```python
from build123d import *

# Parameters (mm, degrees)
ESBO_O1_W                = 23
ESBO_O1_H                = 38
ESBO_O1_W_2              = 15
ESBO_O1_H_2              = 30
RESSALTO_EXTRUS_O1_DEPTH = 3
CHANFRO1_SIZE            = 2
CHANFRO1_SIZE2           = 2.14473742
CHANFRO1_PART_2_SIZE     = 2
CHANFRO1_PART_2_SIZE2    = 2.14473742
CHANFRO1_PART_3_SIZE     = 2
CHANFRO1_PART_3_SIZE2    = 2.14473742
CHANFRO1_PART_4_SIZE     = 2
CHANFRO1_PART_4_SIZE2    = 2.14473742


with BuildPart() as part:
    # Esboço1 → Ressalto-extrusão1 (new body)
    with BuildSketch(Plane.XY):
        Rectangle(ESBO_O1_W, ESBO_O1_H)
        Rectangle(ESBO_O1_W_2, ESBO_O1_H_2, mode=Mode.SUBTRACT)
    extrude(amount=RESSALTO_EXTRUS_O1_DEPTH)

    # Chanfro1
    chanfro1_edges = [part.edges().sort_by_distance(p)[0] for p in [
        (11.5, 0, 3),
    ]]
    chanfro1_side = [part.faces().sort_by_distance(p)[0] for p in [
        (11.5, 0, 1.5),
    ]]
    chamfer(chanfro1_edges, length=CHANFRO1_SIZE, length2=CHANFRO1_SIZE2, reference=chanfro1_side[0])

    # Chanfro1 part 2
    chanfro1_part_2_edges = [part.edges().sort_by_distance(p)[0] for p in [
        (0, 19, 3),
    ]]
    chanfro1_part_2_side = [part.faces().sort_by_distance(p)[0] for p in [
        (0, 19, 1.5),
    ]]
    chamfer(chanfro1_part_2_edges, length=CHANFRO1_PART_2_SIZE, length2=CHANFRO1_PART_2_SIZE2, reference=chanfro1_part_2_side[0])

    # Chanfro1 part 3
    chanfro1_part_3_edges = [part.edges().sort_by_distance(p)[0] for p in [
        (-11.5, 0, 3),
    ]]
    chanfro1_part_3_side = [part.faces().sort_by_distance(p)[0] for p in [
        (-11.5, 0, 1.5),
    ]]
    chamfer(chanfro1_part_3_edges, length=CHANFRO1_PART_3_SIZE, length2=CHANFRO1_PART_3_SIZE2, reference=chanfro1_part_3_side[0])

    # Chanfro1 part 4
    chanfro1_part_4_edges = [part.edges().sort_by_distance(p)[0] for p in [
        (0, -19, 3),
    ]]
    chanfro1_part_4_side = [part.faces().sort_by_distance(p)[0] for p in [
        (0, -19, 1.5),
    ]]
    chamfer(chanfro1_part_4_edges, length=CHANFRO1_PART_4_SIZE, length2=CHANFRO1_PART_4_SIZE2, reference=chanfro1_part_4_side[0])


solid = part.part
```
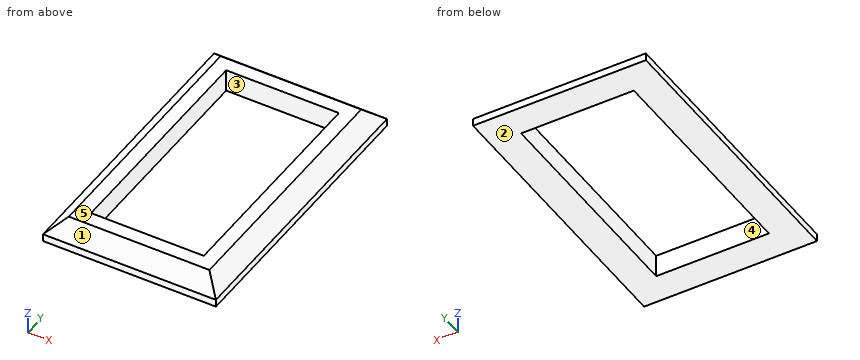
Verification items for the finished model (mm, model axes). Face numbers are marked on the shaded views. A direction names the side the tool comes from. Coordinates: 2 decimals unless noted, no trailing zeros. Loops run counter-clockwise (first coordinate to the right, second up) from the corner with the lowest first, then second, coordinate; pieces in that order, holes last. Notation, with made-up numbers: (20.5, -33) - (45.5, -33) arc R25 ccw to (45.5, -17) - close; hole circle Ø9 at (29.25, -13.5). An arc over 180 degrees is marked (long way). Return JSON: item names as keys, results as strings.
1. Section check C-C, the plane z = 0.4. Record the boundary of the cut face in (x, y).
Established:
{"outline": "(-11.5, -19) - (11.5, -19) - (11.5, 19) - (-11.5, 19) - close; hole (-7.5, -15) - (7.5, -15) - (7.5, 15) - (-7.5, 15) - close"}
2. Mould release check, pull along Y, two halves, no side actions. Record for the marked faces 1, 2 and 3: +Y half, -Y half, draft (parallel to the pull), parting line (faces both ways), or undercut.
Established:
{"face 1": "-Y half", "face 2": "draft", "face 3": "undercut"}
3. Section check D-D, the plane x = -8.75. Record the boundary of the cut face in (y, z).
Established:
{"outline": "(-19, 0) - (19, 0) - (19, 1) - (16.86, 3) - (-16.86, 3) - (-19, 1) - close"}
4. Section check B-B, the plane x = -6. Record the boundary of the cut face in (y, z).
Established:
{"outline": "(-19, 0) - (-15, 0) - (-15, 3) - (-16.86, 3) - (-19, 1) - close; (15, 0) - (19, 0) - (19, 1) - (16.86, 3) - (15, 3) - close"}
5. Section check A-A, the plane y = -13.5. Record the boundary of the cut face in (x, z), then the cut area to 3 significant figures.
Established:
{"outline": "(-11.5, 0) - (-7.5, 0) - (-7.5, 3) - (-9.36, 3) - (-11.5, 1) - close; (7.5, 0) - (11.5, 0) - (11.5, 1) - (9.36, 3) - (7.5, 3) - close", "area": "19.7 mm2"}
6. Go/stop test with a flat-tipped pin: pin 1 (1 mm diameter, centred on x = -5.5, z = 2, fed in from -Y). Record where the tip stops, or that it passes through.
Established:
{"pin 1": "stops at y = -18.46"}
7. Tool access check on the marked faces 4 and 5. Record the directions out of +Z, -Z, +X, -X, +Y, -Y that give a thin tool (end or side, any length) a straight path to the whole face; none if there is none.
Established:
{"face 4": "+Z, -Z", "face 5": "+Z, +X, -X, +Y, -Y"}
8. Thickness scan on L1, parallel to Y at x = -4.25, z = 0.85; L2, parallel to X at y = -6, z = 0.8; L3, parallel to X at y = -14.5, z = 1.1. Record the ranges inside material, lowest first.
Established:
{"L1": "y = -19 to -15, 15 to 19", "L2": "x = -11.5 to -7.5, 7.5 to 11.5", "L3": "x = -11.39 to -7.5, 7.5 to 11.39"}
